```python
from build123d import *

# Parameters (mm, degrees)
SKETCH_219_W       = 2.5
SKETCH_219_H       = 5.25
EXTRUDE_2643_DEPTH = 2


with BuildPart() as part:
    # Sketch 219 → Revolve 1 (revolve)
    with BuildSketch(Plane.XY, mode=Mode.PRIVATE) as revolve_1_sk:
        with BuildLine():
            ThreePointArc((11.2, 4.8), (10.2627417, 7.0627417), (8, 8))
            Line((8, 8), (8, 0))
            Line((8, 0), (11.2, 0))
            Line((11.2, 0), (11.2, 0.68))
            Line((11.2, 0.68), (11.2, 4.8))
        make_face()
        Polygon((0, 11), (0, 0), (1, 0), (1, 5.25), (3.5, 5.25), (3.5, 0), (5, 0), (5, 11), align=None)
        with BuildLine():
            ThreePointArc((8, 8), (7.121320344, 10.121320344), (5, 11))
            Line((5, 11), (5, 0))
            Line((5, 0), (8, 0))
            Line((8, 0), (8, 8))
        make_face()
        with Locations((2.25, 2.625)):
            Rectangle(SKETCH_219_W, SKETCH_219_H)
    revolve(revolve_1_sk.sketch.rotate(Axis((0, 0, 0), (1, 0, 0)), 90), axis=Axis((0, 0, 0), (1, 0, 0)))

    # Sketch 1503 → Extrude 2643 (add, symmetric)
    with BuildSketch(Plane.XY):
        with BuildLine():
            ThreePointArc((11.2, 4.4), (29.338267199, 10.995701086), (45.2, 0))
            Line((45.2, 0), (11.2, 0))
            Line((11.2, 0), (11.2, 4.4))
        make_face()
        with BuildLine():
            Line((31.263463773, 0), (11.2, 0))
            Line((11.2, 0), (11.2, -3.914978255))
            ThreePointArc((11.2, -3.914978255), (22.080678837, -6.30816882), (31.263463773, 0))
        make_face()
        Polygon((38.912013935, 0), (35.248695767, 0), (35.248695767, -11.07), (38.912013935, -4.32), align=None)
        Polygon((35.248695767, 0), (31.263463773, 0), (32.498964702, -1.197255299), (32.498964702, -9.797255299), (35.248695767, -11.07), align=None)
        Polygon((42.083014277, -1.2), (42.083014277, 0), (40.307542508, 0), (40.307542508, -6.49), align=None)
        Polygon((40.307542508, 0), (38.912013935, 0), (38.912013935, -4.32), (40.307542508, -6.49), align=None)
        Polygon((42.083014277, -1.2), (45.2, 0), (42.083014277, 0), align=None)
    extrude(amount=EXTRUDE_2643_DEPTH, both=True)

    # Sketch 16 → Revolve 2 (revolve)
    with BuildSketch(Plane.XY):
        with BuildLine():
            ThreePointArc((8, 8), (7.121320344, 10.121320344), (5, 11))
            Line((5, 11), (5, 0))
            Line((5, 0), (8, 0))
            Line((8, 0), (8, 8))
        make_face()
    revolve(axis=Axis((0, 0, 0), (1, 0, 0)))


solid = part.part
```
Work out the finished part from the listing and answer in its coordinate system (mm). A direction names the side the tool comes from. Round coordinates to 2 decimals unless told otherwise and drop trailing zeros. Loops run counter-clockwise (first coordinate to the right, second up) from the corner with the lowest first, then second, coordinate; pieces in that order, holes last. Notation, with made-up numbers: (-38.75, -15) -> (-33.75, -15) arc R34 cw to (-33.75, 23) -> close; hole circle Ø8 at (19.5, 27.25). An arc over 180 degrees is marked (long way). Write each question's results on one line, items separated by ' | '. Start each with the question number.
1. Section D-D (x = 38) is taken. Determine the outline of the cut face in (y, z), plus the area to 3 significant figures.
2. Section C-C (x = 25.5) is taken. Determine the outline of the cut face in (y, z).
3. Section B-B (z = 0) is taken. Determine the outline of the cut face in (x, y).
4. Find the intervals of material crossed by probe 1 along Z at (x, y) = (35, -2); probe 2 along X at (y, z) = (-0.5, 8.25); probe 3 along X at (y, z) = (8.25, 0.25), in increasing order. Write a range as from..to.
5. Given pin 1 Ø5 at (y, z) = (7.5, 6.5) entering from +X; pin 2 Ø5 at (x, z) = (5.5, -4) entering from +Y; pin 3 Ø10 at (x, z) = (13.5, 6) entering from -Y; pin 4 Ø2 at (x, y) = (19.5, -9) entering from -Z, each flat-ended and moving along its own axis, determine where each tip first touches the part or whether it passes through.
6. For a pull along X with two mould halves and no side action, classify faces 4 (the face through (0, 0, 0)), 5 (the face through (28, 3, -2)), 6 (the face through (37.055, -7.742, 0.028)) as +X half, -X half, draft (parallel to the pull), parting line (faces both ways), or undercut.
7. A tool of negligible diameter and unlimited length cuts with its end or side. For faces 1 (the face through (33.855, -10.425, 0.028)), 2 (the face through (28, 3, 2)), 3 (the face through (43.62, -0.61, 0.03)), from which of +Z, -Z, +X, -X, +Y, -Y can it reach the whole face along a straight path? Write none if from no direction.
8. Section A-A (x = 4.5) is taken. Determine the outline of the cut face in (y, z).
Evaluation:
1) outline: (-6, -2) -> (7.83, -2) -> (7.83, 2) -> (-6, 2) -> close | area: 55.3 mm2
2) outline: (-5.17, -2) -> (11.14, -2) -> (11.14, 2) -> (-5.17, 2) -> close
3) outline: (0, -11) -> (5, -11) arc R3 ccw to (8, -8) arc R3.2 ccw to (11.2, -4.8) -> (11.2, -3.91) arc R14 ccw to (31.26, 0) -> (32.5, -1.2) -> (32.5, -9.8) -> (35.25, -11.07) -> (38.91, -4.32) -> (40.31, -6.49) -> (42.08, -1.2) -> (45.2, 0) arc R21 ccw to (11.2, 4.4) -> (11.2, 4.8) arc R3.2 ccw to (8, 8) arc R3 ccw to (5, 11) -> (0, 11) -> close
4) probe 1: z = -2..2 | probe 2: x = 0..7.99 | probe 3: x = 0..7.99, 15.96..37.32
5) pin 1: stops at x = 9.83 | pin 2: stops at y = 10.89 | pin 3: stops at y = -7.01 | pin 4: passes through
6) face 4: -X half | face 5: draft | face 6: undercut
7) face 1: +Z, -Z, -Y | face 2: +Z, +X, +Y, -Y | face 3: +Z, -Z, +X, -Y
8) outline: circle Ø22 at (0, 0)
